Verification items for the finished model (mm, model axes). Face numbers are marked on the shaded views. A direction names the side the tool comes from. Coordinates: 2 decimals unless noted, no trailing zeros. Order: outer loops, then holes, each group sorted by start corner. A loop starts at its lowest first (then second) coordinate and runs counter-clockwise, first axis right, second up. Notation, with made-up numbers: (14, 81.5) - (34, 81.5) arc R26 ccw to (34, 114.5) - close; hole circle Ø8 at (73.25, -35). An arc over 180 degrees is marked (long way). Answer as CSV lines item,"result". Start each with the question number.
1. Material ranges on L1, parallel to X at y = 0.85, z = -3; L2, parallel to X at y = 2, z = -19; L3, parallel to Z at x = 3, y = 0.9, recorded low to high. Write a range as [from, to].
2. Go/stop test with flat-tipped pins: pin 1 (2.5 mm diameter, centred on x = 3, z = -3, fed in from -Y); pin 2 (0.8 mm diameter, centred on x = 22, y = 2.5, fed in from -Z); pin 3 (1.6 mm diameter, centred on y = 2.5, z = -14.5, fed in from -X); pin 4 (3 mm diameter, centred on x = 5.5, y = 4, fed in from -Z). Record where each tip stops, or that it passes through.
3. Section check C-C (y = 0.75). Record the cut outline in (x, z).
4. Section check D-D (y = 4.5). Record the cut outline in (x, z).
5. Set-up check for the marked faces 1, 2, 3 and 4: record each of +Z, -Z, +X, -X, +Y, -Y from which the full face is reachable in a straight line by a thin tool's end or side.
6. Section check B-B (x = 3). Record the cut outline in (y, z).
7. Section check A-A (z = -29). Record the cut outline in (x, y), and give its area (3 significant figures).
from build123d import *

# Parameters (mm, degrees)
SKETCH1_W                 = 42
SKETCH1_H                 = 32
PCB_DEPTH                 = 1.6
MOUNT_HOLE_1_DEPTH        = 53.825751296
MOUNT_HOLE_1_DEPTH_BACK   = 53.825751296
SKETCH2_R                 = 1.5
MOUNT_HOLE_2_DEPTH        = 53.825751296
MOUNT_HOLE_2_DEPTH_BACK   = 53.825751296
SKETCH3_R                 = 1.5
MOUNT_HOLE_3_DEPTH        = 53.825751296
MOUNT_HOLE_3_DEPTH_BACK   = 53.825751296
SKETCH4_R                 = 1.5
MOUNT_HOLE_4_DEPTH        = 53.825751296
MOUNT_HOLE_4_DEPTH_BACK   = 53.825751296
SKETCH5_R                 = 1.5
PROBE_CONNECTOR_XH_START  = 1.6
SKETCH6_W                 = 7
SKETCH6_H                 = 10
PROBE_CONNECTOR_XH_DEPTH  = 6
SIGNAL_CONNECTOR_PH_START = 1.6
SKETCH7_W                 = 6
SKETCH7_H                 = 9
SIGNAL_CONNECTOR_PH_DEPTH = 6
SIGNAL_IC_START           = 1.6
SKETCH8_W                 = 8
SKETCH8_H                 = 8
SIGNAL_IC_DEPTH           = 1.5


with BuildPart() as part:
    # Sketch1 → PCB (new body)
    with BuildSketch(Plane(origin=(0, 0, 0), x_dir=(1, 0, 0), z_dir=(0, 1, 0))):
        with Locations((21, 16)):
            Rectangle(SKETCH1_W, SKETCH1_H)
    extrude(amount=PCB_DEPTH)

    # Sketch2 → Mount_hole_1 (cut, two sides: drawn at the far end of the back side and taken through both)
    with BuildSketch(Plane(origin=(0, 0, 0), x_dir=(1, 0, 0), z_dir=(0, 1, 0)).offset(-MOUNT_HOLE_1_DEPTH_BACK)):
        with Locations(Location((3, 3, 0), (0, 0, 270))):
            Circle(SKETCH2_R)
    extrude(amount=MOUNT_HOLE_1_DEPTH + MOUNT_HOLE_1_DEPTH_BACK, mode=Mode.SUBTRACT)

    # Sketch3 → Mount_hole_2 (cut, two sides: drawn at the far end of the back side and taken through both)
    with BuildSketch(Plane(origin=(0, 0, 0), x_dir=(1, 0, 0), z_dir=(0, 1, 0)).offset(-MOUNT_HOLE_2_DEPTH_BACK)):
        with Locations(Location((39, 3, 0), (0, 0, 270))):
            Circle(SKETCH3_R)
    extrude(amount=MOUNT_HOLE_2_DEPTH + MOUNT_HOLE_2_DEPTH_BACK, mode=Mode.SUBTRACT)

    # Sketch4 → Mount_hole_3 (cut, two sides: drawn at the far end of the back side and taken through both)
    with BuildSketch(Plane(origin=(0, 0, 0), x_dir=(1, 0, 0), z_dir=(0, 1, 0)).offset(-MOUNT_HOLE_3_DEPTH_BACK)):
        with Locations(Location((3, 29, 0), (0, 0, 270))):
            Circle(SKETCH4_R)
    extrude(amount=MOUNT_HOLE_3_DEPTH + MOUNT_HOLE_3_DEPTH_BACK, mode=Mode.SUBTRACT)

    # Sketch5 → Mount_hole_4 (cut, two sides: drawn at the far end of the back side and taken through both)
    with BuildSketch(Plane(origin=(0, 0, 0), x_dir=(1, 0, 0), z_dir=(0, 1, 0)).offset(-MOUNT_HOLE_4_DEPTH_BACK)):
        with Locations(Location((39, 29, 0), (0, 0, 270))):
            Circle(SKETCH5_R)
    extrude(amount=MOUNT_HOLE_4_DEPTH + MOUNT_HOLE_4_DEPTH_BACK, mode=Mode.SUBTRACT)

    # Sketch6 → Probe_connector_XH (add)
    with BuildSketch(Plane(origin=(0, 0, 0), x_dir=(1, 0, 0), z_dir=(0, 1, 0)).offset(PROBE_CONNECTOR_XH_START)):
        with Locations((5.5, 16)):
            Rectangle(SKETCH6_W, SKETCH6_H)
    extrude(amount=PROBE_CONNECTOR_XH_DEPTH)

    # Sketch7 → Signal_connector_PH (add)
    with BuildSketch(Plane(origin=(0, 0, 0), x_dir=(1, 0, 0), z_dir=(0, 1, 0)).offset(SIGNAL_CONNECTOR_PH_START)):
        with Locations((36, 15.5)):
            Rectangle(SKETCH7_W, SKETCH7_H)
    extrude(amount=SIGNAL_CONNECTOR_PH_DEPTH)

    # Sketch8 → Signal_IC (add)
    with BuildSketch(Plane(origin=(0, 0, 0), x_dir=(1, 0, 0), z_dir=(0, 1, 0)).offset(SIGNAL_IC_START)):
        with Locations((21, 16)):
            Rectangle(SKETCH8_W, SKETCH8_H)
    extrude(amount=SIGNAL_IC_DEPTH)


solid = part.part
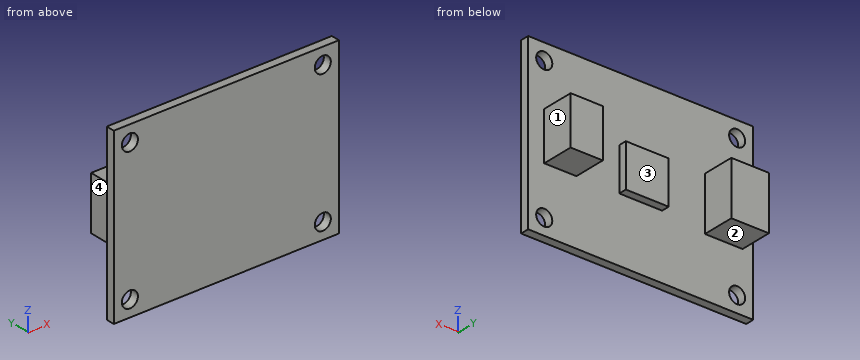
Evaluation:
1,L1,"x = [0, 1.5], [4.5, 37.5], [40.5, 42]"
1,L2,"x = [2, 9], [17, 25], [33, 39]"
1,L3,"z = [-32, -30.5], [-27.5, -4.5], [-1.5, 0]"
2,pin 1,"passes through"
2,pin 2,"stops at z = -20"
2,pin 3,"stops at x = 2"
2,pin 4,"stops at z = -21"
3,outline,"(0, -32) - (42, -32) - (42, 0) - (0, 0) - close; hole circle Ø3 at (3, -29); hole circle Ø3 at (3, -3); hole circle Ø3 at (39, -29); hole circle Ø3 at (39, -3)"
4,outline,"(2, -21) - (9, -21) - (9, -11) - (2, -11) - close; (33, -20) - (39, -20) - (39, -11) - (33, -11) - close"
5,face 1,"+Z, -Z, +X, +Y"
5,face 2,"-Z, +X, -X, +Y"
5,face 3,"+Z, -Z, +Y"
5,face 4,"+Z, -Z, -X, +Y"
6,outline,"(0, -32) - (1.6, -32) - (1.6, -30.5) - (0, -30.5) - close; (0, -27.5) - (1.6, -27.5) - (1.6, -21) - (7.6, -21) - (7.6, -11) - (1.6, -11) - (1.6, -4.5) - (0, -4.5) - close; (0, -1.5) - (1.6, -1.5) - (1.6, 0) - (0, 0) - close"
7,outline,"(0, 0) - (1.5, 0) - (1.5, 1.6) - (0, 1.6) - close; (4.5, 0) - (37.5, 0) - (37.5, 1.6) - (4.5, 1.6) - close; (40.5, 0) - (42, 0) - (42, 1.6) - (40.5, 1.6) - close"
7,area,"57.6 mm²"
